For this review, take the finished solid that the model builds, in its own axes (mm). A direction names the side the tool comes from. Coordinates: 2 decimals unless noted, no trailing zeros. Order: outer loops, then holes, each group sorted by start corner. A loop starts at its lowest first (then second) coordinate and runs counter-clockwise, first axis right, second up. Notation, with made-up numbers: (35, 9) -> (90, 9) arc R12 ccw to (90, 14) -> close; hole circle Ø6 at (72, 9). An arc over 180 degrees is marked (long way). Write item = value, one per line. Start each with the question number.
1) Wall thickness on probe 1 along Y at (x, z) = (-46, 1.7); probe 2 along Y at (x, z) = (0, 0.85); probe 3 along Y at (x, z) = (-21.5, 1.75): over which ranges is each line inside the solid? List them lowest first. Write a range as [from, to].
2) Draft analysis for pull direction X (two halves, no side actions). For faces 1 (the face through (19, 28, 1)), 2 (the face through (-21, 0, 2)), 3 (the face through (-40, -3.068, 1)), 4 (the face through (-57.98, -27.53, 0.99)), state which applies: +X half, -X half, draft (parallel to the pull), parting line (faces both ways), or undercut.
3) Machinability: for faces 5 (the face through (-23, -29, 1)), 6 (the face through (18, -29, 1)), which of the approach directions +Z, -Z, +X, -X, +Y, -Y give a long, thin tool a straight path to every point of the face, cutting with its end or side? Answer none if there is none.
4) Consider section A-A on x = -16. Give the boundary of the cut face in (y, z), and give its area (3 significant figures).
5) Consider section B-B on z = 1.25. State how many separate pieces and enclosed holes the cut face has, and give its area (3 significant figures).
6) Consider section C-C on y = 16. Give the boundary of the cut face in (x, z), and give its area (3 significant figures).
7) Consider section D-D on x = -3. Give the boundary of the cut face in (y, z), and give its area (3 significant figures).
Autodesk Inventor part; units mm, degrees
ref_plane "YZ Plane" through (0, 0, 0) normal (1, 0, 0) x (0, 1, 0)
ref_plane "XZ Plane" through (0, 0, 0) normal (0, 1, 0) x (-1, 0, 0)
ref_plane "XY Plane" through (0, 0, 0) normal (0, 0, 1) x (1, 0, 0)
sketch "Sketch1" plane through (0, 0, 0) normal (0, 0, 1) x (1, 0, 0)
  circle A0 centre (0, 0) radius 15
  circle A1 centre (16, 16) radius 1.5
  circle A2 centre (-16, 16) radius 1.5
  circle A3 centre (-16, -16) radius 1.5
  circle A4 centre (16, -16) radius 1.5
  line L0 (20, -18) -> (20, 18)
  line L1 (18, 20) -> (-18, 20)
  line L2 (-60.0198, 26.9978) -> (-59.9853, -20.0189)
  line L3 (-18, -20) -> (18, -20)
  line L4 (-57.0198, 30) -> (-15.022, 30)
  line L5 (-14.978, -30) -> (-56.9802, -30)
  line L6 (-59.9802, -27.0022) -> (-60.0198, 26.9978)
  line L7 (-57.9798, -27.5) -> (12.0202, -27.5) construction
  line L8 (-56.4798, -29) -> (10.5202, -29)
  line L9 (10.5202, -26) -> (-56.4798, -26)
  arc A5 (-56.4798, -26) -> (-56.4798, -29) centre (-56.4798, -27.5) ccw
  arc A6 (10.5202, -29) -> (10.5202, -26) centre (10.5202, -27.5) ccw
  arc A7 (-59.9802, -27.0022) -> (-56.9802, -30) centre (-56.9802, -27) ccw
  arc A8 (-57.0198, 30) -> (-60.0198, 26.9978) centre (-57.0198, 27) ccw
  line L10 (-58.0202, 27.5) -> (11.9798, 27.5) construction
  line L11 (-56.5202, 26) -> (10.4798, 26)
  line L12 (10.4798, 29) -> (-56.5202, 29)
  arc A9 (-56.5202, 29) -> (-56.5202, 26) centre (-56.5202, 27.5) ccw
  arc A10 (10.4798, 26) -> (10.4798, 29) centre (10.4798, 27.5) ccw
  line L13 (20, -18) -> (20, 18)
  line L14 (-14.978, -30) -> (20, -30)
  line L15 (20, -30) -> (20, -18)
  line L16 (20, -30) -> (-56.9802, -30)
  line L17 (-60.0198, -29) -> (-60.0198, 27)
  line L18 (-57.0198, 30) -> (20, 30)
  line L19 (20, 30) -> (20, -30)
  point P0 (0, 0)
  point P1 (-60.0198, 26.9811)
  point P2 (-59.978, -30)
  point P3 (-22.9798, -27.5)
  point P4 (-23.0202, 27.5)
  dimension "d11" = 70
  dimension "d12" = 3
  dimension "d13" = 2.5
  dimension "d15" = 3.5
  dimension "d16" = 3
  dimension "d17" = 3
  dimension "d18" = 3
  dimension "d19" = 70
  dimension "d21" = 3.5
  dimension "d26" = 30
  dimension "d27" = 60
  dimension "d28" = 2.5
  dimension "d29" = 45
  dimension "d30" = 45
  dimension "d31" = 60
  dimension "d32" = 79.9853
  dimension "d33" = 80.0198
extrude "Extrusion1" add sketch "Sketch1" along normal blind 2
fillet "Fillet1" radius 5 2 edges at (20, -30, 1) (20, 30, 1)
sketch "Sketch4" plane through (0, 0, 2) normal (0, 0, 1) x (1, 0, 0)
  line L0 (-21.95, -0.0183) -> (-57.05, -0.0183) construction
  line L1 (-25, 3.0317) -> (-54, 3.0317)
  line L2 (-54, -3.0683) -> (-25, -3.0683)
  arc A0 (-25, -3.0683) -> (-25, 3.0317) centre (-25, -0.0183) ccw
  arc A1 (-54, 3.0317) -> (-54, -3.0683) centre (-54, -0.0183) ccw
  circle A2 centre (0, 0) radius 15
  line L3 (-60.0198, 26.9978) -> (-59.9802, -27.0022)
  point P0 (0, 0)
  point P1 (-39.5, -0.0183)
  dimension "d34" = 6.1
  dimension "d35" = 25
  dimension "d36" = 6
extrude "Extrusion2" cut sketch "Sketch4" against normal through all contours A0 L2 A1 L1
equation "\"d18\" = d12"
equation "\"d19\" = d11"
equation "\"d21\" = d15"
equation "\"d30\" = d29"
properties part number "X-motor-holder-offset"
Answer sheet:
q1.probe_1 = [-30, -29], [-26, -3.07], [3.03, 26], [29, 30]
q1.probe_2 = [-30, -29], [-26, -15], [15, 26], [29, 30]
q1.probe_3 = [-30, -29], [-26, 26], [29, 30]
q2.face_1 = +X half
q2.face_2 = draft
q2.face_3 = undercut
q2.face_4 = undercut
q3.face_5 = +Z, -Z
q3.face_6 = +Z, -Z, +X, -Y
q4.outline = (-30, 0) -> (-29, 0) -> (-29, 2) -> (-30, 2) -> close; (-26, 0) -> (-17.5, 0) -> (-17.5, 2) -> (-26, 2) -> close; (-14.5, 0) -> (14.5, 0) -> (14.5, 2) -> (-14.5, 2) -> close; (17.5, 0) -> (26, 0) -> (26, 2) -> (17.5, 2) -> close; (29, 0) -> (30, 0) -> (30, 2) -> (29, 2) -> close
q4.area = 96.0 mm2
q5.separate_pieces = 1
q5.enclosed_holes = 8
q5.area = 3,430 mm2
q6.outline = (-60.01, 0) -> (-17.5, 0) -> (-17.5, 2) -> (-60.01, 2) -> close; (-14.5, 0) -> (14.5, 0) -> (14.5, 2) -> (-14.5, 2) -> close; (17.5, 0) -> (20, 0) -> (20, 2) -> (17.5, 2) -> close
q6.area = 148 mm2
q7.outline = (-30, 0) -> (-29, 0) -> (-29, 2) -> (-30, 2) -> close; (-26, 0) -> (-14.7, 0) -> (-14.7, 2) -> (-26, 2) -> close; (14.7, 0) -> (26, 0) -> (26, 2) -> (14.7, 2) -> close; (29, 0) -> (30, 0) -> (30, 2) -> (29, 2) -> close
q7.area = 49.2 mm2
